Source: CAD feature listing. Evaluate the final solid. Frame: model axes, mm. Face numbers are marked on the shaded views. Coordinates: 2 decimals unless noted, no trailing zeros. Write each loop counter-clockwise with the first axis right and the second up, starting at its lowest first coordinate (ties: lowest second). Pieces come first, ordered by that corner, then holes. Notation, with made-up numbers: (80.25, 43.5) -> (101.25, 43.5) arc R30 ccw to (101.25, 71.5) -> close; hole circle Ø1 at (-10, -13.75). An arc over 180 degrees is marked (long way). Write item = value, one per line.
from build123d import *

# Parameters (mm, degrees)
SKETCH1_W                  = 241.3
SKETCH1_H                  = 38.1
BOSS_EXTRUDE1_DEPTH        = 3.175
SKETCH2_R                  = 2.54
CUT_EXTRUDE1_DEPTH         = 3.175
LPATTERN1_COUNT            = 16
LPATTERN1_PITCH            = 12.7
SKETCHED_START             = -120.65
SKETCHED_BEND2_OUTLINE_W   = 3.175
SKETCHED_BEND2_OUTLINE_H   = 38.1
SKETCHED_BEND2_DEPTH       = 25.4
SKETCHED_START_2           = -94.869557784
SKETCHED_BEND2_2_OUTLINE_W = 26.397512257
SKETCHED_BEND2_2_OUTLINE_H = 38.1
SKETCHED_BEND2_2_OUTLINE_R = 2.54
SKETCHED_BEND2_2_DEPTH     = 2.794557784
SKETCHED_START_3           = -95.25
SKETCHED_BEND2_3_OUTLINE_W = 26.397512257
SKETCHED_BEND2_3_OUTLINE_H = 38.1
SKETCHED_BEND2_3_OUTLINE_R = 2.54
SKETCHED_BEND2_3_DEPTH     = 3.9116
SKETCHED_START_4           = -20
SKETCHED_BEND2_4_DEPTH     = 40
SKETCHED_START_5           = -19.05
SKETCHED_BEND3_DEPTH       = 38.1
SKETCHED_BEND3_2_DEPTH     = 38.1
SKETCH28_R                 = 2.372260046
CUT_EXTRUDE2_DEPTH         = 10.922
LPATTERN2_COUNT            = 2
LPATTERN2_PITCH            = 12.7


with BuildPart() as part:
    # Sketch1 → Boss-Extrude1 (new body)
    with BuildSketch(Plane(origin=(0, 0, 0), x_dir=(1, 0, 0), z_dir=(0, 1, 0))):
        Rectangle(SKETCH1_W, SKETCH1_H)
    extrude(amount=BOSS_EXTRUDE1_DEPTH)

    # Sketch2 → Cut-Extrude1 (cut)
    with BuildSketch(Plane(origin=(0, 3.175, 0), x_dir=(1, 0, 0), z_dir=(0, 1, 0))):
        with Locations(Location((-110.49, 0, 0), (0, 0, 270))):
            Circle(SKETCH2_R)
    cut_extrude1 = extrude(amount=-CUT_EXTRUDE1_DEPTH, mode=Mode.SUBTRACT)

    # LPattern1: Cut-Extrude1 ×16
    with Locations(*[(i * LPATTERN1_PITCH, 0, 0) for i in range(1, LPATTERN1_COUNT)]):
        add(cut_extrude1, mode=Mode.SUBTRACT)

    # Sketched Bend2: read off the stored shape, not the designer's step
    # Sketched Bend2 outline → Sketched Bend2 (cut)
    with BuildSketch(Plane.YZ.offset(SKETCHED_START)):
        with Locations((1.5875, 0)):
            Rectangle(SKETCHED_BEND2_OUTLINE_W, SKETCHED_BEND2_OUTLINE_H)
    extrude(amount=SKETCHED_BEND2_DEPTH, mode=Mode.SUBTRACT)

    # Sketched Bend2 2 outline → Sketched Bend2 2 (add)
    with BuildSketch(Plane.YZ.offset(SKETCHED_START_2)):
        with Locations((16.373756129, 0)):
            Rectangle(SKETCHED_BEND2_2_OUTLINE_W, SKETCHED_BEND2_2_OUTLINE_H)
        with Locations((6.712512257, 0)):
            Circle(SKETCHED_BEND2_2_OUTLINE_R, mode=Mode.SUBTRACT)
        with Locations((19.412512257, 0)):
            Circle(SKETCHED_BEND2_2_OUTLINE_R, mode=Mode.SUBTRACT)
    extrude(amount=SKETCHED_BEND2_2_DEPTH)

    # Sketched Bend2 3 outline → Sketched Bend2 3 (add)
    with BuildSketch(Plane.YZ.offset(SKETCHED_START_3)):
        with Locations((16.373756129, 0)):
            Rectangle(SKETCHED_BEND2_3_OUTLINE_W, SKETCHED_BEND2_3_OUTLINE_H)
        with Locations((6.712512257, 0)):
            Circle(SKETCHED_BEND2_3_OUTLINE_R, mode=Mode.SUBTRACT)
        with Locations((19.412512257, 0)):
            Circle(SKETCHED_BEND2_3_OUTLINE_R, mode=Mode.SUBTRACT)
    extrude(amount=SKETCHED_BEND2_3_DEPTH)

    # Sketched Bend2 4 outline → Sketched Bend2 4 (cut)
    with BuildSketch(Plane.XY.offset(SKETCHED_START_4)):
        with BuildLine():
            ThreePointArc((-91.3384, 0), (-94.104318885, 1.145681115), (-95.25, 3.9116))
            Line((-95.25, 3.9116), (-95.25, 0))
            Line((-95.25, 0), (-91.3384, 0))
        make_face()
        with BuildLine():
            Line((-92.075, 29.572512257), (-92.075, 3.9116))
            ThreePointArc((-92.075, 3.9116), (-91.859254855, 3.390745145), (-91.3384, 3.175))
            Line((-91.3384, 3.175), (-91.3384, 29.572512257))
            Line((-91.3384, 29.572512257), (-92.075, 29.572512257))
        make_face()
    extrude(amount=SKETCHED_BEND2_4_DEPTH, mode=Mode.SUBTRACT)

    # Sketched Bend3: read off the stored shape, not the designer's step
    # Sketched Bend3 outline → Sketched Bend3 (cut)
    with BuildSketch(Plane.XY.offset(SKETCHED_START_5)):
        with BuildLine():
            Line((120.65, 3.175), (95.180018799, 3.175))
            ThreePointArc((95.180018799, 3.175), (93.830319942, 0.896479843), (91.3384, 0))
            Line((91.3384, 0), (120.65, 0))
            Line((120.65, 0), (120.65, 3.175))
        make_face()
    extrude(amount=SKETCHED_BEND3_DEPTH, mode=Mode.SUBTRACT)

    # Sketched Bend3 2 outline → Sketched Bend3 2 (add)
    with BuildSketch(Plane.XY.offset(SKETCHED_START_5)):
        with BuildLine():
            Line((95.25, 29.572512257), (92.075, 29.572512257))
            Line((92.075, 29.572512257), (92.075, 3.9116))
            ThreePointArc((92.075, 3.9116), (91.859254855, 3.390745145), (91.3384, 3.175))
            Line((91.3384, 3.175), (95.180018799, 3.175))
            ThreePointArc((95.180018799, 3.175), (95.232465398, 3.541641581), (95.25, 3.9116))
            Line((95.25, 3.9116), (95.25, 29.572512257))
        make_face()
    extrude(amount=SKETCHED_BEND3_2_DEPTH)

    # Sketch28 → Cut-Extrude2 (cut)
    with BuildSketch(Plane.ZY.offset(-92.075)):
        with Locations(Location((0, 19.412512257, 0), (0, 0, 270))):
            Circle(SKETCH28_R)
    cut_extrude2 = extrude(amount=-CUT_EXTRUDE2_DEPTH, mode=Mode.SUBTRACT)

    # LPattern2: Cut-Extrude2 ×2
    with Locations(*[(0, -i * LPATTERN2_PITCH, 0) for i in range(1, LPATTERN2_COUNT)]):
        add(cut_extrude2, mode=Mode.SUBTRACT)


solid = part.part
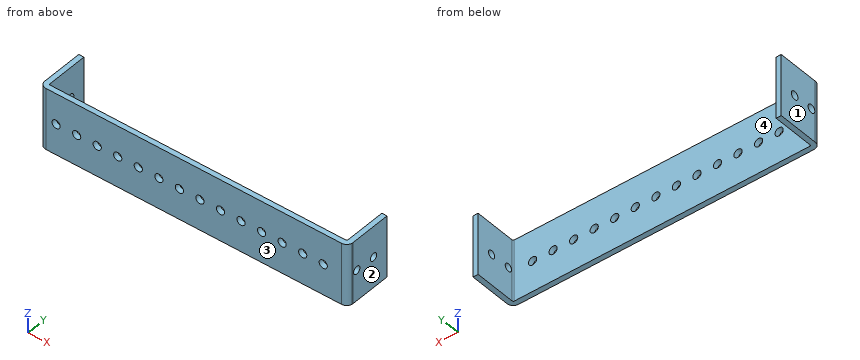
1) Cut plane A-A, the plane x = -72.39. Output: boundary loops of the cut face in (y, z) (3 decimals).
Answer block:
outline = (0, -19.05) -> (3.175, -19.05) -> (3.175, -2.54) -> (0, -2.54) -> close; (0, 2.54) -> (3.175, 2.54) -> (3.175, 19.05) -> (0, 19.05) -> close
2) Material intervals for probe 1 along X at (y, z) = (22, -14) (3 decimals); probe 2 along Z at (x, y) = (67.31, 1.35); probe 3 along Y at (x, z) = (46, -6) (3 decimals), sorted ascending. Write a range as [from, to].
Answer block:
probe_1 = [-95.25, -92.075], [92.075, 95.25]
probe_2 = [-19.05, -2.54], [2.54, 19.05]
probe_3 = [0, 3.175]
3) Pull-direction query (X, two-part tool) for the marked faces 1, 2, 3 and 4; classes: +X half, -X half, draft (parallel to the pull), parting line (faces both ways), or undercut.
Answer block:
face_1 = -X half
face_2 = +X half
face_3 = draft
face_4 = undercut
4) Cut plane C-C, the plane z = 15.5. Output: boundary loops of the cut face in (x, y) (3 decimals), and give its area (3 significant figures).
Answer block:
outline = (-95.25, 3.912) arc R3.912 ccw to (-91.338, 0) -> (91.338, 0) arc R3.912 ccw to (95.25, 3.912) -> (95.25, 29.573) -> (92.075, 29.573) -> (92.075, 3.912) arc R0.737 cw to (91.338, 3.175) -> (-91.338, 3.175) arc R0.737 cw to (-92.075, 3.912) -> (-92.075, 29.573) -> (-95.25, 29.573) -> close
area = 766 mm2
5) First-contact query: pin 1 Ø6.5 at (x, z) = (-72.39, 0) entering from -Y; pin 2 Ø1 at (x, z) = (51.5, 13.5) entering from +Y (3 decimals). Flat tips, straight axial feed; report the tip coordinate or a pass-through.
Answer block:
pin_1 = 0
pin_2 = 3.175
6) Cut plane B-B, the plane y = 12. Output: boundary loops of the cut face in (x, z) (3 decimals).
Answer block:
outline = (-95.25, -19.05) -> (-92.075, -19.05) -> (-92.075, 19.05) -> (-95.25, 19.05) -> close; (92.075, -19.05) -> (95.25, -19.05) -> (95.25, 19.05) -> (92.075, 19.05) -> close
